Work out the finished part from the listing and answer in its coordinate system (mm). Face numbers are marked on the shaded views. A direction names the side the tool comes from. Coordinates: 2 decimals unless noted, no trailing zeros. Loops run counter-clockwise (first coordinate to the right, second up) from the corner with the lowest first, then second, coordinate; pieces in that order, holes last.
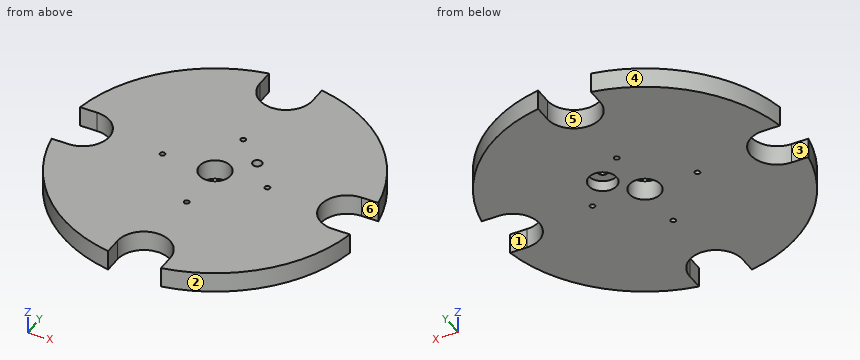
```python
from build123d import *

# Parameters (mm, degrees)
ESQUISSE1_R             = 195
ESQUISSE1_R_2           = 20
BASE_EXTRUSION_DEPTH    = 26
ENL_V_MAT_EXTRU_1_DEPTH = 277.994584785
PER_AGE1_D              = 6.6
ESQUISSE5_R             = 6
ENL_V_MAT_EXTRU_2_DEPTH = 273.789295978
ESQUISSE6_R             = 18
ENL_V_MAT_EXTRU_3_DEPTH = 14


with BuildPart() as part:
    # Esquisse1 → Base-Extrusion (new body)
    with BuildSketch(Plane.XY):
        Circle(ESQUISSE1_R)
        with Locations(Location((0, 0, 0), (0, 0, 180))):
            Circle(ESQUISSE1_R_2, mode=Mode.SUBTRACT)
    extrude(amount=BASE_EXTRUSION_DEPTH)

    # Esquisse2 → Enlèv. mat.-Extru.1 (cut, through all)
    with BuildSketch(Plane.XY.offset(26)):
        with BuildLine():
            Line((170, 34), (192.013020392, 34))
            ThreePointArc((192.013020392, 34), (195, 0), (192.013020392, -34))
            Line((192.013020392, -34), (170, -34))
            ThreePointArc((170, -34), (136, 0), (170, 34))
        make_face()
        with BuildLine():
            Line((34, -170), (34, -192.013020392))
            ThreePointArc((34, -192.013020392), (0, -195), (-34, -192.013020392))
            Line((-34, -192.013020392), (-34, -170))
            ThreePointArc((-34, -170), (0, -136), (34, -170))
        make_face()
        with BuildLine():
            Line((-170, -34), (-192.013020392, -34))
            ThreePointArc((-192.013020392, -34), (-195, 0), (-192.013020392, 34))
            Line((-192.013020392, 34), (-170, 34))
            ThreePointArc((-170, 34), (-136, 0), (-170, -34))
        make_face()
        with BuildLine():
            Line((-34, 170), (-34, 192.013020392))
            ThreePointArc((-34, 192.013020392), (0, 195), (34, 192.013020392))
            Line((34, 192.013020392), (34, 170))
            ThreePointArc((34, 170), (0, 136), (-34, 170))
        make_face()
    extrude(amount=-ENL_V_MAT_EXTRU_1_DEPTH, mode=Mode.SUBTRACT)

    # Perçage1 (through all)
    with Locations(Plane.XY.offset(26)):
        with Locations((0, 67.5), (67.5, 0), (0, -67.5), (-67.5, 0)):
            Hole(PER_AGE1_D / 2)

    # Esquisse5 → Enlèv. mat.-Extru.2 (cut, through all)
    with BuildSketch(Plane.XY.offset(26)):
        with Locations((35.355339059, 35.355339059)):
            Circle(ESQUISSE5_R)
    extrude(amount=-ENL_V_MAT_EXTRU_2_DEPTH, mode=Mode.SUBTRACT)

    # Esquisse6 → Enlèv. mat.-Extru.3 (cut)
    with BuildSketch(Plane(origin=(0, 0, 0), x_dir=(-1, 0, 0), z_dir=(0, 0, -1))):
        with Locations((-35.355339059, 35.355339059)):
            Circle(ESQUISSE6_R)
    extrude(amount=-ENL_V_MAT_EXTRU_3_DEPTH, mode=Mode.SUBTRACT)


solid = part.part
```
1. Determine the mould class of the marked faces 4, 5 and 6 for opening direction X: released by +X, released by -X, zero draft, split by the parting line, or undercut.
2. A cutting plane is placed at A-A, the plane y = 153. Give the vertices of the cut face in (x, z).
3. A cutting plane is placed at C-C, the plane z = 19.75. Give the vertices of the cut face in (x, y), then the cut area to 3 significant figures.
4. Each of these flat-tipped pins is pushed along its axis until it touches: P1, Ø1, axis at x = 61.5, z = 11, coming from the +Y side; P2, Ø11, axis at x = -180, z = 17.5, coming from the -Y side; P3, Ø6, axis at y = 120, z = 6, coming from the -X side; P4, Ø6, axis at x = 0, y = -67.5, coming from the +Z side. Where does it stop, or does it pass through?
5. A cutting plane is placed at B-B, the plane x = -146.5. Give the vertices of the cut face in (y, z), then the cut area to 3 significant figures.
6. For the marked faces 1, 2 and 3, determine the directions among +Z, -Z, +X, -X, +Y, -Y from which every point of the face is accessible in a straight line to the end or side of a thin tool.
7. A cutting plane is placed at D-D, the plane y = 48. Give the vertices of the cut face in (x, z), then the cut area to 3 significant figures.
8. Straight lines are drawn through the part: probe 1 along Y at (x, z) = (0, 10.5); probe 2 along X at (y, z) = (-15.5, 24.5); probe 3 along Y at (x, z) = (-5, 5). For each, find the intervals that lie inside material, in ascending order.
Answers below:
1. face 4: released by -X
1. face 5: undercut
1. face 6: zero draft
2. outline: (-120.9, 0) - (-29.44, 0) - (-29.44, 26) - (-120.9, 26) - close; (29.44, 0) - (120.9, 0) - (120.9, 26) - (29.44, 26) - close
3. outline: (-192.01, -34) arc R195 ccw to (-34, -192.01) - (-34, -170) arc R34 cw to (34, -170) - (34, -192.01) arc R195 ccw to (192.01, -34) - (170, -34) arc R34 cw to (170, 34) - (192.01, 34) arc R195 ccw to (34, 192.01) - (34, 170) arc R34 cw to (-34, 170) - (-34, 192.01) arc R195 ccw to (-192.01, 34) - (-170, 34) arc R34 cw to (-170, -34) - close; hole circle Ø6.6 at (-67.5, 0); hole circle Ø40 at (0, 0); hole circle Ø6.6 at (0, -67.5); hole circle Ø6.6 at (0, 67.5); hole circle Ø12 at (35.36, 35.36); hole circle Ø6.6 at (67.5, 0)
3. area: 104,000 mm2
4. P1: stops at y = 185.21
4. P2: stops at y = -87.03
4. P3: stops at x = -156
4. P4: passes through
5. outline: (-128.7, 0) - (-24.57, 0) - (-24.57, 26) - (-128.7, 26) - close; (24.57, 0) - (128.7, 0) - (128.7, 26) - (24.57, 26) - close
5. area: 5,410 mm2
6. face 1: +Z, -Z, +X
6. face 2: +Z, -Z, +X, -Y
6. face 3: +Z, -Z, -X
7. outline: (-189, 0) - (22.54, 0) - (22.54, 14) - (48.17, 14) - (48.17, 0) - (189, 0) - (189, 26) - (-189, 26) - close
7. area: 9,470 mm2
8. probe 1: y = -136 to -70.8, -64.2 to -20, 20 to 64.2, 70.8 to 136
8. probe 2: x = -139.74 to -12.64, 12.64 to 139.74
8. probe 3: y = -136.37 to -19.36, 19.36 to 136.37
